Study the drawing (mm; zero at the part's minimum x, y, z) and answer. Coordinates: 2 decimals unless noted, no trailing zeros. Loops run counter-clockwise (first coordinate to the right, second up) from the corner with the lowest first, then second, coordinate; pieces in that order, holes last. Notation, with made-up numbers: (51.25, -39) -> (109.25, -39) arc R23 cw to (109.25, -31) -> close; hole circle Ø6 at (83, -19.75). An arc over 180 degrees is marked (long way). Answer as CSV lines item,"result".
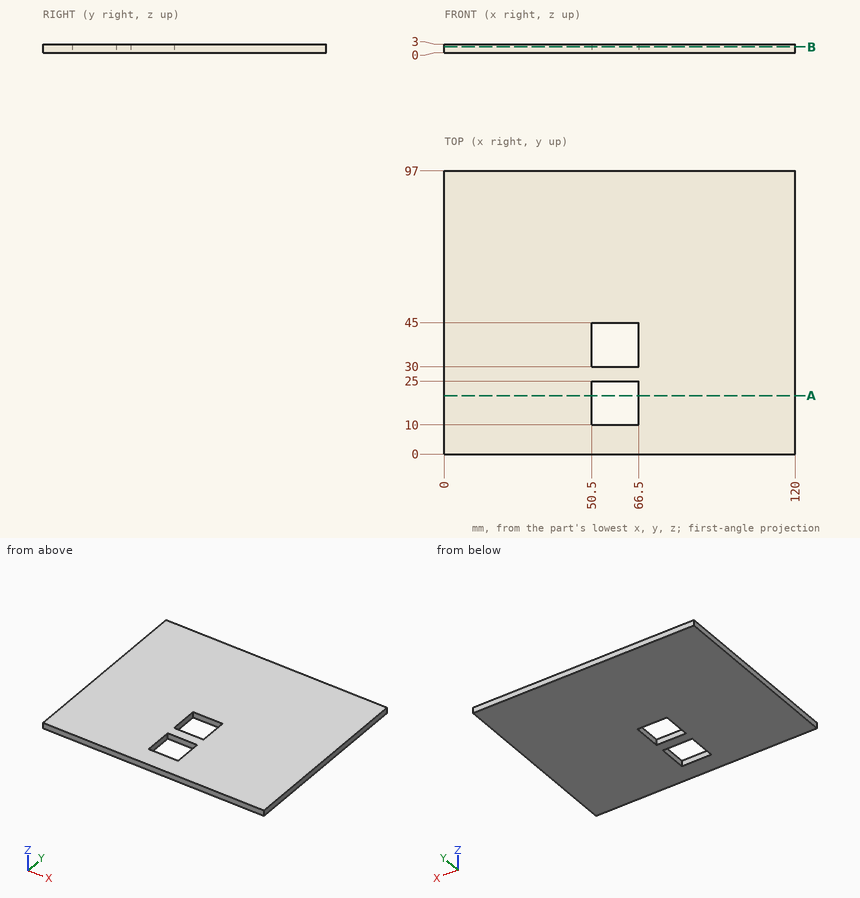
Q1. A cutting plane is placed at A-A, the plane y = 20. Write down the section's boundary in (x, z).
Results:
outline,"(0, 0) -> (50.5, 0) -> (50.5, 3) -> (0, 3) -> close; (66.5, 0) -> (120, 0) -> (120, 3) -> (66.5, 3) -> close"
Q2. Given pin 1 Ø5 at (x, y) = (55.5, 44) entering from -Z, flat-ended and moving along its own axis, determine where the tip first touches the part or whether it passes through.
Results:
pin 1,"stops at z = 0"
Q3. A cutting plane is placed at B-B, the plane z = 2. Write down the section's boundary in (x, y).
Results:
outline,"(0, 0) -> (120, 0) -> (120, 97) -> (0, 97) -> close; hole (50.5, 10) -> (66.5, 10) -> (66.5, 25) -> (50.5, 25) -> close; hole (50.5, 30) -> (66.5, 30) -> (66.5, 45) -> (50.5, 45) -> close"
Q4. Find the intervals of material crossed by probe 1 along Y at (x, z) = (55, 0.75); probe 2 along X at (y, z) = (23, 0.5), in increasing order. Write a range as [from, to].
Results:
probe 1,"y = [0, 10], [25, 30], [45, 97]"
probe 2,"x = [0, 50.5], [66.5, 120]"
